from build123d import *

# Parameters (mm, degrees)
SKETCH1_W           = 1000
SKETCH1_H           = 500
BOSS_EXTRUDE1_DEPTH = 25.4
SKETCH2_R           = 20
BOSS_EXTRUDE2_DEPTH = 750


with BuildPart() as part:
    # Sketch1 → Boss-Extrude1 (new body)
    with BuildSketch(Plane.XY):
        Rectangle(SKETCH1_W, SKETCH1_H)
    extrude(amount=BOSS_EXTRUDE1_DEPTH)

    # Sketch2 → Boss-Extrude2 (add)
    with BuildSketch(Plane.XY):
        with Locations((460, 210)):
            Circle(SKETCH2_R)
        with Locations((460, -210)):
            Circle(SKETCH2_R)
        with Locations((-460, -210)):
            Circle(SKETCH2_R)
        with Locations((-460, 210)):
            Circle(SKETCH2_R)
    extrude(amount=-BOSS_EXTRUDE2_DEPTH)


solid = part.part
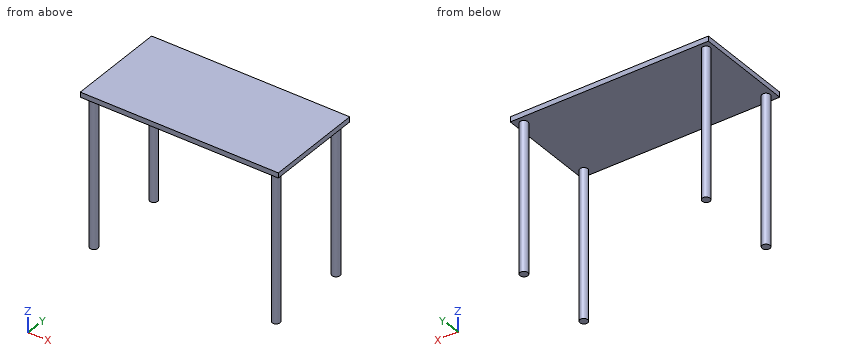
Can you work these out from the model? Positions are in its coordinate system, mm. Round coordinates to 2 decimals unless told otherwise and drop trailing zeros. Write each loop counter-clockwise with the first axis right and the second up, starting at its lowest first coordinate (ties: lowest second). Pieces come first, ordered by that corner, then holes. Notation, with made-up numbers: (56.25, 20) -> (108.25, 20) arc R9 ccw to (108.25, 34) -> close; hole circle Ø9 at (41, -1). An arc over 180 degrees is marked (long way). Use one line per item in the form item = value. Start each with the question number.
Q1. Imagine slicing it at A-A (y = 210). Please give me the cut outline in (x, z).
Q2. If I drill on probe 1 along X at (y, z) = (-211.5, -525.5); probe 2 along Y at (x, z) = (-457, -653.5); probe 3 along Z at (x, y) = (-397, 216), over which ranges is the centre line in solid material (lowest first)? Write a range as [from, to].
Q3. I'm going to push a flat-ended pin straight in: P1, Ø8, axis at x = -65, y = 7.5, coming from the -Z side. Where does the tip first touch, or does it pass through?
Q4. Imagine slicing it at C-C (z = -330.5). Please give me the cut outline in (x, y), then the cut area to 3 significant figures.
Q5. Imagine slicing it at B-B (x = -460). Please give me the cut outline in (y, z).
Q6. Imagine slicing it at D-D (x = 290.5). Please give me the cut outline in (y, z).
Worked out:
q1.outline = (-500, 0) -> (-480, 0) -> (-480, -750) -> (-440, -750) -> (-440, 0) -> (440, 0) -> (440, -750) -> (480, -750) -> (480, 0) -> (500, 0) -> (500, 25.4) -> (-500, 25.4) -> close
q2.probe_1 = [-479.94, -440.06], [440.06, 479.94]
q2.probe_2 = [-229.77, -190.23], [190.23, 229.77]
q2.probe_3 = [0, 25.4]
q3.P1 = 0
q4.outline = circle Ø40 at (-460, -210); circle Ø40 at (-460, 210); circle Ø40 at (460, -210); circle Ø40 at (460, 210)
q4.area = 5,030 mm^2
q5.outline = (-250, 0) -> (-230, 0) -> (-230, -750) -> (-190, -750) -> (-190, 0) -> (190, 0) -> (190, -750) -> (230, -750) -> (230, 0) -> (250, 0) -> (250, 25.4) -> (-250, 25.4) -> close
q6.outline = (-250, 0) -> (250, 0) -> (250, 25.4) -> (-250, 25.4) -> close
